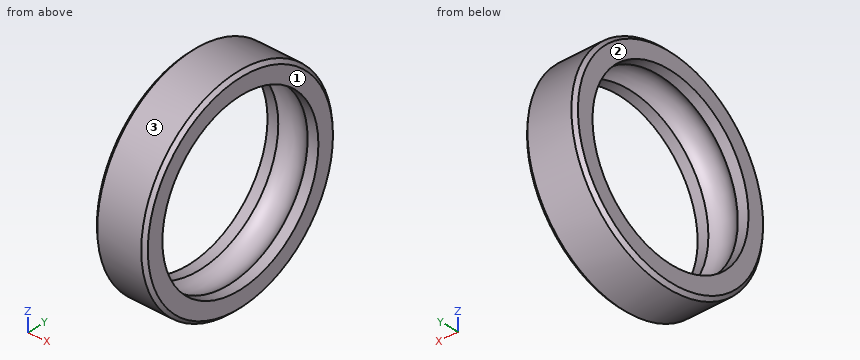
```python
from build123d import *

# Parameters (mm, degrees)
CHAMFER1_SIZE = 2.1


with BuildPart() as part:
    # Sketch1 → Revolve1 (revolve)
    with BuildSketch(Plane.XY):
        with BuildLine():
            Line((-15.5, 65), (15.5, 65))
            Line((15.5, 65), (15.5, 53))
            Line((15.5, 53), (8.94427191, 53))
            ThreePointArc((8.94427191, 53), (0, 57), (-8.94427191, 53))
            Line((-8.94427191, 53), (-15.5, 53))
            Line((-15.5, 53), (-15.5, 65))
        make_face()
    revolve(axis=Axis((-47.365464456, 0, 0), (1, 0, 0)))

    # Chamfer1
    chamfer1_edges = [part.edges().sort_by_distance(p)[0] for p in [
        (15.5, -65, 0),
        (-15.5, -65, 0),
    ]]
    chamfer(chamfer1_edges, length=CHAMFER1_SIZE)


solid = part.part
```
Design review of the part built by this model. Coordinates are the model's own, in mm. Face numbers are marked on the shaded views. Give positions to 0.01 mm unless a question says otherwise; leave off trailing zeros. Write each loop counter-clockwise with the first axis right and the second up, starting at its lowest first coordinate (ties: lowest second). Pieces come first, ordered by that corner, then holes. Notation, with made-up numbers: (58, 65.25) - (78, 65.25) arc R19 ccw to (78, 97.25) - close; hole circle Ø9 at (1, -16). An arc over 180 degrees is marked (long way). Return JSON: item names as keys, results as strings. Group by question number.
(1) To check wall thickness, follow probe 1 along Z at (x, y) = (11, 0); probe 2 along Y at (x, z) = (-5, -38.5); probe 3 along X at (y, z) = (30, -47.5). State the ranges of each line that lie inside material, in increasing order.
(2) We need section A-A, the plane z = 0. Give the boundary of the cut face in (x, y), then the cut area to 3 significant figures.
(3) We need section C-C, the plane x = -11. Give the boundary of the cut face in (y, z), then the cut area to 3 significant figures.
(4) We need section D-D, the plane x = 5. Give the boundary of the cut face in (y, z), then the cut area to 3 significant figures.
(5) Mouldability with a two-part tool opening along X and no side actions: class the marked faces 1, 2 and 3 as +X half, -X half, draft (parallel to the pull), parting line (faces both ways), or undercut.
(6) Insertion check: pin 1 (10 mm diameter, centred on x = 6.5, z = -24.5, fed in from -Y); pin 2 (8 mm diameter, centred on x = -10.5, y = 15.5, fed in from +Z); pin 3 (1 mm diameter, centred on x = 7, y = -47.5, fed in from +Z). Each pin has a flat end and moves straight along its axis. Give the tip position at first contact, or say it passes through.
Reported:
{
 "1": {"probe 1": "z = -65 to -53, 53 to 65", "probe 2": "y = -52.37 to -40.54, 40.54 to 52.37", "probe 3": "x = -15.5 to -4.36, 4.36 to 15.5"},
 "2": {"outline": "(-15.5, -62.9) - (-13.4, -65) - (13.4, -65) - (15.5, -62.9) - (15.5, -53) - (8.94, -53) arc R12 cw to (-8.94, -53) - (-15.5, -53) - close; (-15.5, 53) - (-8.94, 53) arc R12 cw to (8.94, 53) - (15.5, 53) - (15.5, 62.9) - (13.4, 65) - (-13.4, 65) - (-15.5, 62.9) - close", "area": "636 mm2"},
 "3": {"outline": "circle Ø130 at (0, 0); hole circle Ø106 at (0, 0)", "area": "4,450 mm2"},
 "4": {"outline": "circle Ø130 at (0, 0); hole circle Ø111.82 at (0, 0)", "area": "3,450 mm2"},
 "5": {"face 1": "+X half", "face 2": "-X half", "face 3": "draft"},
 "6": {"pin 1": "stops at y = -62.01", "pin 2": "stops at z = 63.97", "pin 3": "stops at z = 44.9"}
}
